```python
from build123d import *

# Parameters (mm, degrees)
ESQUISSE1_R             = 3
BOSS_EXTRU_1_DEPTH      = 20
ESQUISSE2_R             = 2
ENL_V_MAT_EXTRU_1_DEPTH = 44.874821937
CONG_1_R                = 5
D_GAGEMENT_M61_D        = 6.6


with BuildPart() as part:
    # Esquisse1 → Boss.-Extru.1 (new body)
    with BuildSketch(Plane(origin=(0, 0, 0), x_dir=(1, 0, 0), z_dir=(0, 1, 0))):
        with BuildLine():
            Line((30, 0), (-30, 0))
            Line((-30, 0), (-30, 17.468719423))
            ThreePointArc((-30, 17.468719423), (-21.983350692, 24.984343437), (-15, 16.5))
            Line((-15, 16.5), (15, 16.5))
            ThreePointArc((15, 16.5), (21.983350692, 24.984343437), (30, 17.468719423))
            Line((30, 17.468719423), (30, 0))
        make_face()
        with Locations(Location((-22.468719423, 17.468719423, 0), (0, 0, 270))):
            Circle(ESQUISSE1_R, mode=Mode.SUBTRACT)
        with Locations(Location((22.468719423, 17.468719423, 0), (0, 0, 90))):
            Circle(ESQUISSE1_R, mode=Mode.SUBTRACT)
        with BuildLine():
            Line((22, 3), (-22, 3))
            ThreePointArc((-22, 3), (-25, 6), (-22, 9))
            Line((-22, 9), (22, 9))
            ThreePointArc((22, 9), (25, 6), (22, 3))
        make_face(mode=Mode.SUBTRACT)
    extrude(amount=BOSS_EXTRU_1_DEPTH)

    # Esquisse2 → Enlèv. mat.-Extru.1 (cut, through all)
    with BuildSketch(Plane.XY):
        with Locations((0, 8)):
            Circle(ESQUISSE2_R)
    extrude(amount=-ENL_V_MAT_EXTRU_1_DEPTH, mode=Mode.SUBTRACT)

    # Congé1
    cong_1_edges = [part.edges().sort_by_distance(p)[0] for p in [
        (30, 10, 0),
        (-30, 10, 0),
    ]]
    fillet(cong_1_edges, radius=CONG_1_R)

    # Dégagement M61 (through all)
    with Locations(Plane(origin=(0, 20, 0), x_dir=(1, 0, 0), z_dir=(0, 1, 0))):
        with Locations((-22.468719423, 17.468719423), (22.468719423, 17.468719423)):
            Hole(D_GAGEMENT_M61_D / 2)


solid = part.part
```
Model file for the job. Use its own axes, mm. A direction names the side the tool comes from. Coordinates: 2 decimals unless noted, no trailing zeros. Write each loop counter-clockwise with the first axis right and the second up, starting at its lowest first coordinate (ties: lowest second). Pieces come first, ordered by that corner, then holes. Notation, with made-up numbers: (53.5, 23.5) - (107.5, 23.5) arc R20 ccw to (107.5, 29.5) - close; hole circle Ø3 at (27.25, 14). An arc over 180 degrees is marked (long way). One line per question, with ' | ' between items. Start each with the question number.
Q1. Drill centre lines: line 1 (Z direction, x = 0, y = 15); line 2 (Z direction, x = 20.5, y = 15); line 3 (X direction, y = 10.25, z = -14.5). Where is each one in solid material? Low to high. Write a range as [from, to].
Q2. 3-axis set-ups, long thin cutter, end or side, ignore diameter. For faces 4 (the face through (0, 12, -3)), 5 (the face through (30, 10, -11)): which of +Z, -Z, +X, -X, +Y, -Y reach the whole face in a straight line?
Q3. Cut at D-D, the plane y = 4. List the corners of the cut face in (x, z).
Q4. Pin check, flat tip, straight feed: pin 1 (3 mm diameter, centred on x = -0.5, y = 17.5, fed in from -Z). Stop position of the tip, or through.
Q5. Cut at C-C, the plane z = -6. List the corners of the cut face in (x, y), then the cut area to 3 significant figures.
Q6. Cut at B-B, the plane y = 8. List the corners of the cut face in (x, z).
Q7. Cut at A-A, the plane x = 9. List the corners of the cut face in (y, z).
Q8. Pull direction Z, two halves, no side cores. Call faces 1 (the face through (28, 10, -1)), 2 (the face through (0, 12, -9)), 3 (the face through (-30, 10, -11)): pulls with the +Z half, pulls with the -Z half, needs draft (parallel to the pull), parting line crosses it, or undercut.
Answer below:
1) line 1: [-16.5, -9], [-3, 0] | line 2: [-24.74, -20.12], [-14.82, -9], [-3, 0] | line 3: [-30, -23.91], [-21.03, 21.03], [23.91, 30]
2) face 4: +Y, -Y | face 5: +Z, -Z, +X, +Y, -Y
3) outline: (-30, -17.47) arc R7.53 ccw (long way) to (-15, -16.5) - (15, -16.5) arc R7.53 ccw (long way) to (30, -17.47) - (30, -5) arc R5 ccw to (25, 0) - (-25, 0) arc R5 ccw to (-30, -5) - close; hole circle Ø6.6 at (-22.47, -17.47); hole (-22, -9) - (22, -9) arc R3 ccw to (22, -3) - (-22, -3) arc R3 ccw to start; hole circle Ø6.6 at (22.47, -17.47)
4) pin 1: z = -16.5
5) outline: (-30, 0) - (-25, 0) - (-25, 20) - (-30, 20) - close; (25, 0) - (30, 0) - (30, 20) - (25, 20) - close | area: 200 mm^2
6) outline: (-30, -17.47) arc R7.53 ccw (long way) to (-15, -16.5) - (-2, -16.5) - (-2, -9) - (-22, -9) arc R3 cw to (-22, -3) - (-2, -3) - (-2, 0) - (-25, 0) arc R5 ccw to (-30, -5) - close; (2, -16.5) - (15, -16.5) arc R7.53 ccw (long way) to (30, -17.47) - (30, -5) arc R5 ccw to (25, 0) - (2, 0) - (2, -3) - (22, -3) arc R3 cw to (22, -9) - (2, -9) - close; hole circle Ø6.6 at (-22.47, -17.47); hole circle Ø6.6 at (22.47, -17.47)
7) outline: (0, -16.5) - (20, -16.5) - (20, -9) - (0, -9) - close; (0, -3) - (20, -3) - (20, 0) - (0, 0) - close
8) face 1: pulls with the +Z half | face 2: undercut | face 3: needs draft
